Study the drawing (mm; zero at the part's minimum x, y, z) and answer. Coordinates: 2 decimals unless noted, no trailing zeros. Write each loop counter-clockwise with the first axis right and the second up, starting at its lowest first coordinate (ties: lowest second). Pieces come first, ordered by that corner, then holes. Notation, with made-up numbers: (50, 56.5) -> (64, 56.5) arc R38 cw to (64, 94.5) -> close; hole circle Ø7 at (31.5, 39). An arc over 180 degrees is marked (long way). Answer in a Markdown table with one row per item. Add a question column.
Item 1: Section C-C on y = 2 is taken. Write down the section's boundary in (x, z), then the cut area to 3 significant figures.
Item 2: Section A-A on z = 10 is taken. Write down the section's boundary in (x, y), then the cut area to 3 significant figures.
Item 3: For a pull along Z with two mould halves and no side action, classify the marked faces 1, 2 and 3 as +Z half, -Z half, draft (parallel to the pull), parting line (faces both ways), or undercut.
Item 4: Straight lines are drawn through the part: line 1 (X direction, y = 4.5, z = 10); line 2 (X direction, y = 4.5, z = 7.75). For each, find the intervals that lie inside material, in ascending order. Write a range as from..to.
Item 5: Section B-B on x = 10 is taken. Write down the section's boundary in (y, z).
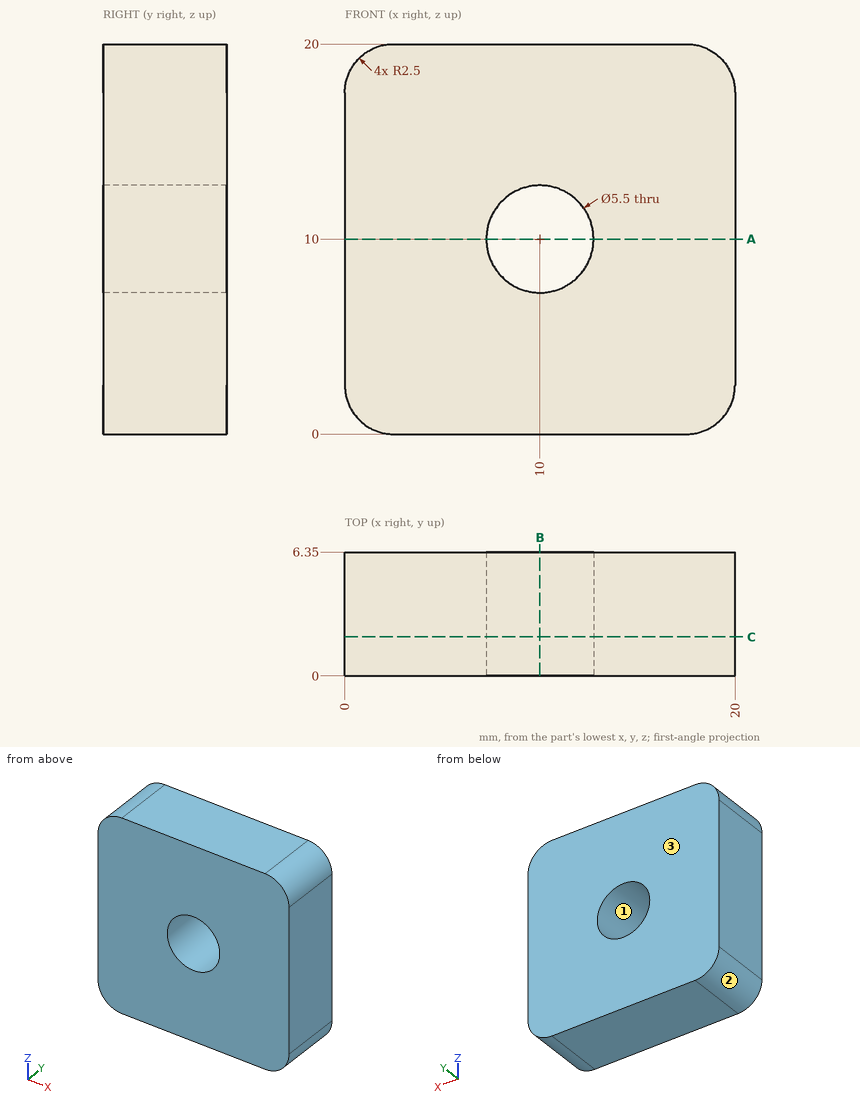
Results below:
| question | item | result |
|---|---|---|
| 1 | outline | (0, 2.5) arc R2.5 ccw to (2.5, 0) -> (17.5, 0) arc R2.5 ccw to (20, 2.5) -> (20, 17.5) arc R2.5 ccw to (17.5, 20) -> (2.5, 20) arc R2.5 ccw to (0, 17.5) -> close; hole circle Ø5.5 at (10, 10) |
| 1 | area | 371 mm2 |
| 2 | outline | (0, 0) -> (7.25, 0) -> (7.25, 6.35) -> (0, 6.35) -> close; (12.75, 0) -> (20, 0) -> (20, 6.35) -> (12.75, 6.35) -> close |
| 2 | area | 92.1 mm2 |
| 3 | face 1 | undercut |
| 3 | face 2 | -Z half |
| 3 | face 3 | draft |
| 4 | line 1 | x = 0..7.25, 12.75..20 |
| 4 | line 2 | x = 0..8.42, 11.58..20 |
| 5 | outline | (0, 0) -> (6.35, 0) -> (6.35, 7.25) -> (0, 7.25) -> close; (0, 12.75) -> (6.35, 12.75) -> (6.35, 20) -> (0, 20) -> close |
